Input: part model. Units: mm. Frame: model coordinates. A direction names the side the tool comes from. Give positions to 0.01 mm unless a question says otherwise; leave off trailing zeros. Loops run counter-clockwise (first coordinate to the right, second up) from the corner with the lowest first, then second, coordinate; pieces in that order, holes last. Notation, with made-up numbers: M -36.75,57 L -25.75,57 A31 ccw -25.75,82 Z; hole C 60.5,20.25 d2. An arc over 180 degrees is marked long. Answer as a JSON object with one key per item and string values. Group by question number.
1) Access query for faces 1 (the cylindrical face through (-37.289, 10.746, 17.696)), 2 (the flat face through (8, 6, 0)), 3 (the flat face through (-41, 2, 0)), 4 (the flat face through (-1, 9, 19.5)). Directions: +Z, -Z, +X, -X, +Y, -Y. A direction counts if a zero-diameter tool reaches every point of the face in a straight line with its end or side. Return the directions, or none.
2) First-contact query: P1, Ø8, axis at x = -21.5, z = -8.5, coming from the +Y side; P2, Ø1.8, axis at x = -36.5, z = 17, coming from the -Y side; P3, Ø3, axis at x = 26, z = -14.5, coming from the -Y side. Flat tips, straight axial feed; report the tip coordinate or a pass-through.
3) Section query A-A on x = -1. Return loops of the section in (y, z), plus the area to 3 significant figures.
4) Section query B-B on y = 8. Return loops of the section in (x, z), plus the area to 3 significant figures.
5) Draft query along Z for faces 5 (the flat face through (-42, 5, 0)), 6 (the flat face through (35, 6, 7.5)), 7 (the flat face through (-31, 6, 0)), 8 (the flat face through (-1, 5, 21.5)). Return one class per face: +Z half, -Z half, draft (parallel to the pull), parting line (faces both ways), or undercut.
6) Ray query, L1, parallel to X at y = 6.75, z = -1.5; L2, parallel to X at y = 2.75, z = 7.5; L3, parallel to Z at x = -20.5, y = 3.75. Return the intervals inside material, ascending.
7) Section query C-C on z = -10.5. Return loops of the section in (x, y), plus the area to 3 significant figures.
8) Section query D-D on z = 6. Return loops of the section in (x, y).
from build123d import *

# Parameters (mm, degrees)
EXTRUDE_1_DEPTH     = 10.5
CUT_EXTRUDE_1_DEPTH = 1
SKETCH_3_R          = 2.5
SKETCH_3_R_2        = 1.65
CUT_EXTRUDE_2_DEPTH = 3.4
SKETCH_4_W          = 78
SKETCH_4_H          = 39
CUT_EXTRUDE_3_DEPTH = 3.5
SKETCH_5_W          = 8
SKETCH_5_H          = 15
CUT_EXTRUDE_4_DEPTH = 48.699580711
SKETCH_6_W          = 16
SKETCH_6_H          = 15
CUT_EXTRUDE_5_DEPTH = 48.699580711
EXTRUDE_2_DEPTH     = 0.5


with BuildPart() as part:
    # 草图1 → 凸台-拉伸1 (new body)
    with BuildSketch(Plane(origin=(0, 0, 0), x_dir=(1, 0, 0), z_dir=(0, 1, 0))):
        with BuildLine():
            Line((-36, 21.5), (36, 21.5))
            ThreePointArc((36, 21.5), (40.242640687, 19.742640687), (42, 15.5))
            Line((42, 15.5), (42, -15.5))
            ThreePointArc((42, -15.5), (40.242640687, -19.742640687), (36, -21.5))
            Line((36, -21.5), (-36, -21.5))
            ThreePointArc((-36, -21.5), (-40.242640687, -19.742640687), (-42, -15.5))
            Line((-42, -15.5), (-42, 15.5))
            ThreePointArc((-42, 15.5), (-40.242640687, 19.742640687), (-36, 21.5))
        make_face()
    extrude(amount=EXTRUDE_1_DEPTH)

    # 草图2 → 切除-拉伸1 (cut)
    with BuildSketch(Plane.XZ):
        with BuildLine():
            Line((36, 20.5), (-36, 20.5))
            ThreePointArc((-36, 20.5), (-39.535533906, 19.035533906), (-41, 15.5))
            Line((-41, 15.5), (-41, -15.5))
            ThreePointArc((-41, -15.5), (-39.535533906, -19.035533906), (-36, -20.5))
            Line((-36, -20.5), (36, -20.5))
            ThreePointArc((36, -20.5), (39.535533906, -19.035533906), (41, -15.5))
            Line((41, -15.5), (41, 15.5))
            ThreePointArc((41, 15.5), (39.535533906, 19.035533906), (36, 20.5))
        make_face()
    extrude(amount=-CUT_EXTRUDE_1_DEPTH, mode=Mode.SUBTRACT)

    # 草图3 → 切除-拉伸2 (cut)
    # profile 1 of 5: a face of its own
    with BuildSketch(Plane(origin=(0, 1, 0), x_dir=(-1, 0, 0), z_dir=(0, -1, 0))):
        with BuildLine():
            Line((-41, 15.5), (-41, -15.5))
            ThreePointArc((-41, -15.5), (-39.535533906, -19.035533906), (-36, -20.5))
            Line((-36, -20.5), (36, -20.5))
            ThreePointArc((36, -20.5), (39.535533906, -19.035533906), (41, -15.5))
            Line((41, -15.5), (41, 15.5))
            ThreePointArc((41, 15.5), (39.535533906, 19.035533906), (36, 20.5))
            Line((36, 20.5), (-36, 20.5))
            ThreePointArc((-36, 20.5), (-39.535533906, 19.035533906), (-41, 15.5))
        make_face()
        with Locations(Location((36, 15.5, 0), (0, 0, 90))):
            Circle(SKETCH_3_R, mode=Mode.SUBTRACT)
        with Locations(Location((36, -15.5, 0), (0, 0, 90))):
            Circle(SKETCH_3_R, mode=Mode.SUBTRACT)
        with Locations(Location((-36, 15.5, 0), (0, 0, 90))):
            Circle(SKETCH_3_R, mode=Mode.SUBTRACT)
        with Locations(Location((-36, -15.5, 0), (0, 0, 90))):
            Circle(SKETCH_3_R, mode=Mode.SUBTRACT)
    # profile 2 of 5: a face of its own
    with BuildSketch(Plane(origin=(0, 1, 0), x_dir=(-1, 0, 0), z_dir=(0, -1, 0))):
        with Locations(Location((36, 15.5, 0), (0, 0, 90))):
            Circle(SKETCH_3_R_2)
    # profile 3 of 5: a face of its own
    with BuildSketch(Plane(origin=(0, 1, 0), x_dir=(-1, 0, 0), z_dir=(0, -1, 0))):
        with Locations(Location((36, -15.5, 0), (0, 0, 90))):
            Circle(SKETCH_3_R_2)
    # profile 4 of 5: a face of its own
    with BuildSketch(Plane(origin=(0, 1, 0), x_dir=(-1, 0, 0), z_dir=(0, -1, 0))):
        with Locations(Location((-36, -15.5, 0), (0, 0, 90))):
            Circle(SKETCH_3_R_2)
    # profile 5 of 5: a face of its own
    with BuildSketch(Plane(origin=(0, 1, 0), x_dir=(-1, 0, 0), z_dir=(0, -1, 0))):
        with Locations(Location((-36, 15.5, 0), (0, 0, 90))):
            Circle(SKETCH_3_R_2)
    extrude(amount=-CUT_EXTRUDE_2_DEPTH, mode=Mode.SUBTRACT)

    # 草图4 → 切除-拉伸3 (cut)
    with BuildSketch(Plane(origin=(0, 10.5, 0), x_dir=(1, 0, 0), z_dir=(0, 1, 0))):
        Rectangle(SKETCH_4_W, SKETCH_4_H)
    extrude(amount=-CUT_EXTRUDE_3_DEPTH, mode=Mode.SUBTRACT)

    # 草图5 → 切除-拉伸4 (cut, through all)
    with BuildSketch(Plane(origin=(0, 7, 0), x_dir=(1, 0, 0), z_dir=(0, 1, 0))):
        with Locations((-35, 0)):
            Rectangle(SKETCH_5_W, SKETCH_5_H)
        with Locations((35, 0)):
            Rectangle(SKETCH_5_W, SKETCH_5_H)
    extrude(amount=-CUT_EXTRUDE_4_DEPTH, mode=Mode.SUBTRACT)

    # 草图6 → 切除-拉伸5 (cut, through all)
    with BuildSketch(Plane(origin=(0, 7, 0), x_dir=(1, 0, 0), z_dir=(0, 1, 0))):
        Rectangle(SKETCH_6_W, SKETCH_6_H)
    extrude(amount=-CUT_EXTRUDE_5_DEPTH, mode=Mode.SUBTRACT)

    # 草图7 → 凸台-拉伸2 (add)
    with BuildSketch(Plane(origin=(0, 10.5, 0), x_dir=(1, 0, 0), z_dir=(0, 1, 0))):
        with BuildLine():
            Line((42, -15.5), (42, 15.5))
            ThreePointArc((42, 15.5), (40.242640687, 19.742640687), (36, 21.5))
            Line((36, 21.5), (-36, 21.5))
            ThreePointArc((-36, 21.5), (-40.242640687, 19.742640687), (-42, 15.5))
            Line((-42, 15.5), (-42, -15.5))
            ThreePointArc((-42, -15.5), (-40.242640687, -19.742640687), (-36, -21.5))
            Line((-36, -21.5), (36, -21.5))
            ThreePointArc((36, -21.5), (40.242640687, -19.742640687), (42, -15.5))
        make_face()
        with BuildLine():
            Line((-33, -19.5), (33, -19.5))
            ThreePointArc((33, -19.5), (37.242640687, -17.742640687), (39, -13.5))
            Line((39, -13.5), (39, 13.5))
            ThreePointArc((39, 13.5), (37.242640687, 17.742640687), (33, 19.5))
            Line((33, 19.5), (-33, 19.5))
            ThreePointArc((-33, 19.5), (-37.242640687, 17.742640687), (-39, 13.5))
            Line((-39, 13.5), (-39, -13.5))
            ThreePointArc((-39, -13.5), (-37.242640687, -17.742640687), (-33, -19.5))
        make_face(mode=Mode.SUBTRACT)
    extrude(amount=EXTRUDE_2_DEPTH)


solid = part.part
Output:
{
 "1": {"face 1": "+Y", "face 2": "+Y, -Y", "face 3": "-Y", "face 4": "none"},
 "2": {"P1": "stops at y = 7", "P2": "stops at y = 1", "P3": "stops at y = 4.4"},
 "3": {"outline": "M 0,-21.5 L 11,-21.5 L 11,-19.5 L 7,-19.5 L 7,-7.5 L 4.4,-7.5 L 4.4,-20.5 L 0,-20.5 Z; M 0,20.5 L 4.4,20.5 L 4.4,7.5 L 7,7.5 L 7,19.5 L 11,19.5 L 11,21.5 L 0,21.5 Z", "area": "97.6 mm^2"},
 "4": {"outline": "M -42,-15.5 A6 ccw -36,-21.5 L 36,-21.5 A6 ccw 42,-15.5 L 42,15.5 A6 ccw 36,21.5 L -36,21.5 A6 ccw -42,15.5 Z; hole M -39,-19.5 L 39,-19.5 L 39,19.5 L -39,19.5 Z", "area": "539 mm^2"},
 "5": {"face 5": "draft", "face 6": "undercut", "face 7": "undercut", "face 8": "+Z half"},
 "6": {"L1": "x = -42 to -39, -31 to -8, 8 to 31, 39 to 42", "L2": "x = -42 to -41, 41 to 42", "L3": "z = -21.5 to -20.5, 20.5 to 21.5"},
 "7": {"outline": "M -42,0 L -41,0 L -41,4.4 L 41,4.4 L 41,0 L 42,0 L 42,11 L 39,11 L 39,7 L -39,7 L -39,11 L -42,11 Z", "area": "251 mm^2"},
 "8": {"outline": "M -42,0 L -41,0 L -41,4.4 L -39,4.4 L -39,11 L -42,11 Z; M -31,4.4 L -8,4.4 L -8,7 L -31,7 Z; M 8,4.4 L 31,4.4 L 31,7 L 8,7 Z; M 39,4.4 L 41,4.4 L 41,0 L 42,0 L 42,11 L 39,11 Z"}
}
